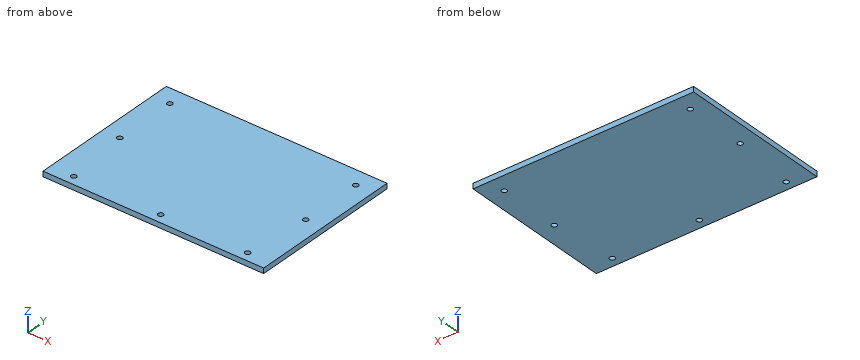
```python
from build123d import *

# Parameters (mm, degrees)
SKETCH_1_W          = 127
SKETCH_1_H          = 92
EXTRUDE_1_DEPTH     = 3
SKETCH_2_R          = 1.5
CUT_EXTRUDE_1_DEPTH = 79.468146403
SKETCH_3_R          = 1.5
CUT_EXTRUDE_2_DEPTH = 79.468146403
SKETCH_4_W          = 127
SKETCH_4_H          = 3.2
CUT_EXTRUDE_3_DEPTH = 10


with BuildPart() as part:
    # 草图1 → 凸台-拉伸1 (new body)
    with BuildSketch(Plane.XY):
        Rectangle(SKETCH_1_W, SKETCH_1_H)
    extrude(amount=EXTRUDE_1_DEPTH)

    # 草图2 → 切除-拉伸1 (cut, through all)
    with BuildSketch(Plane.XY.offset(3)):
        with Locations((0, -37.5)):
            Circle(SKETCH_2_R)
        with Locations((50, -37.5)):
            Circle(SKETCH_2_R)
        with Locations((-50, -37.5)):
            Circle(SKETCH_2_R)
    extrude(amount=-CUT_EXTRUDE_1_DEPTH, mode=Mode.SUBTRACT)

    # 草图3 → 切除-拉伸2 (cut, through all)
    with BuildSketch(Plane.XY.offset(3)):
        with Locations((-53.5, 36)):
            Circle(SKETCH_3_R)
        with Locations((53.5, 36)):
            Circle(SKETCH_3_R)
        with Locations((-53.5, 0)):
            Circle(SKETCH_3_R)
        with Locations((53.5, 0)):
            Circle(SKETCH_3_R)
    extrude(amount=-CUT_EXTRUDE_2_DEPTH, mode=Mode.SUBTRACT)

    # 草图4 → 切除-拉伸3 (cut)
    with BuildSketch(Plane(origin=(0, 0, 0), x_dir=(-1, 0, 0), z_dir=(0, 0, -1))):
        with Locations((0, -44.4)):
            Rectangle(SKETCH_4_W, SKETCH_4_H)
    extrude(amount=-CUT_EXTRUDE_3_DEPTH, mode=Mode.SUBTRACT)


solid = part.part
```
Input: part model. Units: mm. Frame: model coordinates. Give positions to 0.01 mm unless a question says otherwise; leave off trailing zeros. Loops run counter-clockwise (first coordinate to the right, second up) from the corner with the lowest first, then second, coordinate; pieces in that order, holes last. Notation, with made-up numbers: (9.25, 23.5) -> (66.25, 23.5) arc R21 cw to (66.25, 45.5) -> close; hole circle Ø5 at (12, -28.75). An arc over 180 degrees is marked (long way). Use a Markdown table: item, result.
Q1. Section query B-B, the plane y = 0. Return the cut outline in (x, z).
Entries:
| item | result |
|---|---|
| outline | (-63.5, 0) -> (-55, 0) -> (-55, 3) -> (-63.5, 3) -> close; (-52, 0) -> (52, 0) -> (52, 3) -> (-52, 3) -> close; (55, 0) -> (63.5, 0) -> (63.5, 3) -> (55, 3) -> close |
Q2. Ray query, probe 1 along Y at (x, z) = (53.5, 1.7); probe 2 along X at (y, z) = (-36.5, 2.8); probe 3 along Y at (x, z) = (-53, 0.9). Return the intervals inside material, ascending. Write a range as from..to.
Entries:
| item | result |
|---|---|
| probe 1 | y = -42.8..-1.5, 1.5..34.5, 37.5..46 |
| probe 2 | x = -63.5..-51.12, -48.88..-1.12, 1.12..48.88, 51.12..63.5 |
| probe 3 | y = -42.8..-1.41, 1.41..34.59, 37.41..46 |
Q3. Section query A-A, the plane x = 50. Return the cut outline in (y, z).
Entries:
| item | result |
|---|---|
| outline | (-42.8, 0) -> (-39, 0) -> (-39, 3) -> (-42.8, 3) -> close; (-36, 0) -> (46, 0) -> (46, 3) -> (-36, 3) -> close |
